Autodesk Inventor part; units mm, degrees
ref_plane "YZ Plane" through (0, 0, 0) normal (1, 0, 0) x (0, 1, 0)
ref_plane "XZ Plane" through (0, 0, 0) normal (0, 1, 0) x (-1, 0, 0)
ref_plane "XY Plane" through (0, 0, 0) normal (0, 0, 1) x (1, 0, 0)
sketch "Sketch1" plane through (0, 0, 0) normal (0, 1, 0) x (-1, 0, 0)
  line L0 (0, 0) -> (0, -11.468)
  line L1 (0, -11.468) -> (7.843, -11.468)
  line L2 (14.3, -5.011) -> (14.3, 10)
  line L3 (12.5, 10) -> (0, 10)
  line L4 (14.3, -5.011) -> (7.843, -11.468)
  line L5 (0, 0) -> (12.5, 0)
  line L6 (12.5, 0) -> (12.5, 10)
  line L7 (0, 20) -> (0, 31.468)
  line L8 (0, 31.468) -> (7.843, 31.468)
  line L9 (14.3, 25.011) -> (14.3, 10)
  line L10 (14.3, 25.011) -> (7.843, 31.468)
  line L11 (0, 20) -> (12.5, 20)
  line L12 (12.5, 20) -> (12.5, 10)
  line L13 (0.2, -11.268) -> (0.2, -0.2)
  line L14 (0.2, -0.2) -> (12.7, -0.2)
  line L15 (12.7, -0.2) -> (12.7, 10)
  line L16 (12.7, 10) -> (12.7, 20.2)
  line L17 (12.7, 20.2) -> (0.2, 20.2)
  line L18 (0.2, 20.2) -> (0.2, 31.268)
  line L19 (0.2, 31.268) -> (7.7602, 31.268)
  line L20 (7.7602, 31.268) -> (14.1, 24.9282)
  line L21 (14.1, 24.9282) -> (14.1, 10)
  line L22 (14.1, 10) -> (14.1, -4.9282)
  line L23 (14.1, -4.9282) -> (7.7602, -11.268)
  line L24 (7.7602, -11.268) -> (0.2, -11.268)
  point P0 (14.3, -11.468)
  point P1 (14.3, 31.468)
  dimension "d0" = 11.468
  dimension "d1" = 14.3
  dimension "d2" = 21.468
  dimension "d3" = 6.457
  dimension "d4" = 6.457
  dimension "d5" = 12.5
  dimension "d8" = 0.2
extrude "Extrusion1" add sketch "Sketch1" along normal blind 20 contours L13 L14 L15 L16 L17 L18 L19 L20 L21 L22 L23 L24
sketch "Sketch2" plane through (-14.1, 0, -4.9282) normal (-1, 0, 0) x (0, 0, 1)
  line L0 (0, 0) -> (29.8563, 0)
  line L1 (29.8563, 0) -> (29.8563, 20)
  line L2 (0, 20) -> (29.8563, 20)
  line L3 (0, 0) -> (0, 20)
  line L4 (0, 20) -> (29.8563, 20)
  line L5 (14.9282, 20) -> (14.9282, 0)
  line L6 (0, 0) -> (29.8563, 0)
  line L7 (29.8563, 0) -> (29.8563, 20)
  line L8 (29.8563, 10) -> (0, 10)
  line L9 (0, 0) -> (0, 20)
  line L10 (8.6782, 16.25) -> (21.1782, 16.25)
  line L11 (21.1782, 16.25) -> (21.1782, 3.75)
  line L12 (21.1782, 3.75) -> (8.6782, 3.75)
  line L13 (8.6782, 3.75) -> (8.6782, 16.25)
  point P0 (4.9282, 0)
  dimension "d9" = 12.5
  dimension "d10" = 12.5
  dimension "d11" = 6.25
  dimension "d12" = 6.25
extrude "Extrusion2" cut sketch "Sketch2" against normal blind 20 contours L12 L13 L8 L5 | L5 L8 L11 L12 | L13 L10 L5 L8 | L5 L10 L11 L8
properties part number "latticeChamberHolderv1"
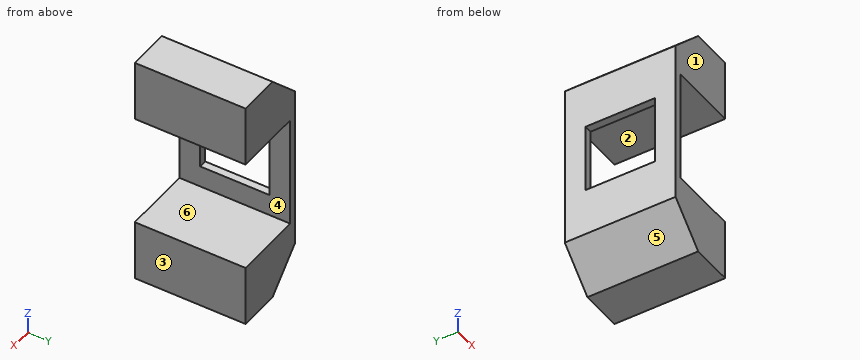
Input: part model. Units: mm. Frame: model coordinates. Face numbers are marked on the shaded views. A direction names the side the tool comes from. Coordinates: 2 decimals unless noted, no trailing zeros. Loops run counter-clockwise (first coordinate to the right, second up) from the corner with the lowest first, then second, coordinate; pieces in that order, holes last. Notation, with made-up numbers: M 51.5,79 L 97.5,79 A29 cw 97.5,100 Z; hole C 83.25,84.5 d6. An arc over 180 degrees is marked long. Answer in a Markdown table with one row per item.
1. Material intervals for line 1 (Z direction, x = -3.25, y = 4.25); line 2 (X direction, y = 17.5, z = 17.5); line 3 (Z direction, x = -8.75, y = 5), sorted ascending.
Response:
| item | result |
|---|---|
| line 1 | z = -11.27 to -0.2, 20.2 to 31.27 |
| line 2 | x = -14.1 to -12.7 |
| line 3 | z = -10.28 to -0.2, 20.2 to 30.28 |
2. Draft query along Z for the marked faces 3, 4, 5 and 6. Return one class per face: pulls with the +Z half, pulls with the -Z half, needs draft (parallel to the pull), parting line crosses it, or undercut.
Response:
| item | result |
|---|---|
| face 3 | needs draft |
| face 4 | undercut |
| face 5 | pulls with the -Z half |
| face 6 | undercut |
3. Section A-A, the plane z = 8. Output: boundary loops of the cut face in (x, y).
Response:
| item | result |
|---|---|
| outline | M -14.1,0 L -12.7,0 L -12.7,3.75 L -14.1,3.75 Z; M -14.1,16.25 L -12.7,16.25 L -12.7,20 L -14.1,20 Z |
4. Section C-C, the plane x = -1. Output: boundary loops of the cut face in (y, z).
Response:
| item | result |
|---|---|
| outline | M 0,-11.27 L 20,-11.27 L 20,-0.2 L 0,-0.2 Z; M 0,20.2 L 20,20.2 L 20,31.27 L 0,31.27 Z |
5. First-contact query: pin 1 (0.7 mm diameter, centred on x = -13, y = 10, fed in from +Z); pin 2 (6 mm diameter, centred on x = -12, y = 12.5, fed in from +Z); pin 3 (1.5 mm diameter, centred on x = -13.5, y = 13, fed in from -Z). Flat tips, straight axial feed; report the tip coordinate or a pass-through.
Response:
| item | result |
|---|---|
| pin 1 | stops at z = 26.38 |
| pin 2 | stops at z = 30.03 |
| pin 3 | stops at z = -6.28 |
6. Reachability of the marked faces 1 and 2 from +Z, -Z, +X, -X, +Y, -Y: full face, straight path, thin tool, end or side. Return the list, or none.
Response:
| item | result |
|---|---|
| face 1 | +Z, -Z, +X, -X, -Y |
| face 2 | +X, +Y, -Y |
7. Section B-B, the plane y = 14.5. Output: boundary loops of the cut face in (x, z), then the cut area to 3 significant figures.
Response:
| item | result |
|---|---|
| outline | M -14.1,-4.93 L -7.76,-11.27 L -0.2,-11.27 L -0.2,-0.2 L -12.7,-0.2 L -12.7,3.75 L -14.1,3.75 Z; M -14.1,16.25 L -12.7,16.25 L -12.7,20.2 L -0.2,20.2 L -0.2,31.27 L -7.76,31.27 L -14.1,24.93 Z |
| area | 279 mm2 |
8. Section D-D, the plane y = 18.25. Output: boundary loops of the cut face in (x, z).
Response:
| item | result |
|---|---|
| outline | M -14.1,-4.93 L -7.76,-11.27 L -0.2,-11.27 L -0.2,-0.2 L -12.7,-0.2 L -12.7,20.2 L -0.2,20.2 L -0.2,31.27 L -7.76,31.27 L -14.1,24.93 Z |
